For this review, take the finished solid that the model builds, in its own axes (mm). A direction names the side the tool comes from. Round coordinates to 2 decimals unless told otherwise and drop trailing zeros. Write each loop counter-clockwise with the first axis right and the second up, starting at its lowest first coordinate (ties: lowest second). Pieces come first, ordered by that corner, then holes. Notation, with made-up numbers: (-25, 50.5) -> (33, 50.5) arc R9 ccw to (33, 60.5) -> close; hole circle Ø5 at (12.5, 54.25). An arc over 180 degrees is marked (long way). Write each question's results on one line, items separated by ' | '. Start each with the question number.
Item 1: Tool access review of faces 5 (the cylindrical face through (0, -24, -36)), 6 (the flat face through (23, 0, -36)), 7 (the cylindrical face through (23.74, -18.524, -6.783)): name each direction out of +Z, -Z, +X, -X, +Y, -Y from which nothing blocks a thin tool from reaching the whole face with its end or side.
Item 2: Add section B-B (y = 10). State the section outline as (x, z) points.
Item 3: Clearance check with flat-ended pins moving along their axes: pin 1 (4 mm diameter, centred on x = 20, y = -19, fed in from -Z); pin 2 (23 mm diameter, centred on y = 6.5, z = -18.5, fed in from +X). State where each tip first meets the part, or that it passes through.
Item 4: Add section C-C (x = -22). State the section outline as (y, z) points.
Item 5: Add section A-A (z = -45). State the section outline as (x, y) points.
Item 6: Add section D-D (x = -3). State the section outline as (y, z) points.
Item 7: To check wall thickness, follow line 1 along Y through (x, z) = (24.8, -7); line 2 along Y through (x, z) = (24, -23); line 3 along Z through (x, y) = (23.7, -19.5). State the ranges of each line that lie inside material, in increasing order.
Item 8: The part is to be moulded in two halves that separate along X. For faces 1 (the flat face through (-2, -24, -60)), 2 (the flat face through (-25, 0, -30)), 3 (the flat face through (0, 23, -30)), 4 (the cylindrical face through (-7, -24, -31)), say which applies: +X half, -X half, draft (parallel to the pull), parting line (faces both ways), or undercut.
Autodesk Inventor part; units mm, degrees
ref_plane "YZ Plane" through (0, 0, 0) normal (1, 0, 0) x (0, 1, 0)
ref_plane "XZ Plane" through (0, 0, 0) normal (0, 1, 0) x (-1, 0, 0)
ref_plane "XY Plane" through (0, 0, 0) normal (0, 0, 1) x (1, 0, 0)
sketch "スケッチ1" plane through (0, 0, 0) normal (0, 0, 1) x (1, 0, 0)
  line L0 (-25, 25) -> (25, 25)
  line L1 (25, 25) -> (25, -25)
  line L2 (25, -25) -> (-25, -25)
  line L3 (-25, -25) -> (-25, 25)
  line L4 (-23, 23) -> (23, 23)
  line L5 (23, 23) -> (23, -23)
  line L6 (23, -23) -> (-23, -23)
  line L7 (-23, -23) -> (-23, 23)
  point P0 (0, 0)
  dimension "d0" = 23
  dimension "d1" = 25
  dimension "d2" = 50
  dimension "d3" = 46
  dimension "d4" = 46
  dimension "d5" = 50
  dimension "d6" = 23
  dimension "d7" = 25
extrude "押し出し1" add sketch "スケッチ1" against normal blind 60
sketch "スケッチ2" plane through (25, -25, 0) normal (1, 0, 0) x (0, 0, -1)
  line L0 (0, 50) -> (0, 0)
  line L1 (0, 0) -> (60, 0)
  circle A0 centre (15, 35) radius 2
  circle A1 centre (45, 29) radius 2
  point P0 (0, 25)
  dimension "d10" = 4
  dimension "d12" = 30
  dimension "d13" = 15
  dimension "d14" = 6
  dimension "d15" = 29
hole "穴1" at (25, 10, -15) at (25, 4, -45) direction (-1, 0, 0) diameter 4 end through all
sketch "スケッチ3" plane through (25, -25, 0) normal (1, 0, 0) x (0, 0, -1)
  circle A0 centre (15, 35) radius 2
  line L0 (0, 50) -> (60, 50)
  line L1 (8.5, 50) -> (21.5, 50)
  line L2 (21.5, 50) -> (21.5, 14.5)
  line L3 (8.5, 14.5) -> (8.5, 50)
  arc A1 (8.5, 14.5) -> (21.5, 14.5) centre (15, 14.5) ccw
  circle A2 centre (45, 29) radius 2
  point P0 (0, 25)
  dimension "d23" = 35.5
  dimension "d26" = 13
  dimension "d27" = 6.5
  dimension "d28" = 6.5
  dimension "d74" = 30
extrude "押し出し2" cut sketch "スケッチ3" against normal blind 2 contours L0 L2 A1 L3
sketch "スケッチ4" plane through (25, -25, 0) normal (1, 0, 0) x (0, 0, -1)
  line L0 (0, 50) -> (8.5, 50)
  line L1 (21.5, 50) -> (60, 50)
  circle A0 centre (7, 41.5) radius 1
  circle A1 centre (7, 5.5) radius 1
  circle A2 centre (23, 41.5) radius 1
  circle A3 centre (23, 5.5) radius 1
  arc A4 (8.5, 14.5) -> (21.5, 14.5) centre (15, 14.5) ccw
  point P0 (0, 25)
  dimension "d32" = 8.5
  dimension "d33" = 8.5
  dimension "d34" = 36
  dimension "d35" = 36
  dimension "d36" = 16
  dimension "d37" = 16
  dimension "d40" = 2
  dimension "d72" = 8
  dimension "d73" = 8
hole "穴2" at (25, 16.5, -7) at (25, 16.5, -23) at (25, -19.5, -7) at (25, -19.5, -23) direction (-1, 0, 0) diameter 2 depth 2 tip angle 118 counterbore diameter 4 counterbore depth 0.5
sketch "スケッチ5" plane through (-25, -25, 0) normal (0, -1, 0) x (1, 0, 0)
  line L0 (50, 0) -> (0, 0)
  line L1 (0, 0) -> (0, -60)
  circle A0 centre (25, -30) radius 5
  point P0 (25, 0)
  dimension "d48" = 25
  dimension "d49" = 30
  dimension "d50" = 10
hole "穴3" at (0, -25, -30) direction (0, 1, 0) diameter 10 depth 2 tip angle 118
sketch "スケッチ6" plane through (-25, -25, 0) normal (0, -1, 0) x (1, 0, 0)
  circle A0 centre (25, -30) radius 5
  line L0 (0, 0) -> (0, -60)
  circle A1 centre (25, -23) radius 1
  point P0 (25, 0)
  dimension "d58" = 2
  dimension "d60" = 7
  dimension "d61" = 25
hole "穴4" at (0, -25, -23) direction (0, 1, 0) diameter 2 depth 2 tip angle 118
pattern_circular "円形状パターン1" count 8 over 360 about axis through (0, -24, -30) along (0, -1, 0) of "穴4"
properties part number "Arm_Bracket_2"
Responses:
1) face 5: -Y | face 6: +Z, -Z | face 7: +X
2) outline: (-25, -60) -> (-23, -60) -> (-23, -17) -> (-25, -17) -> close; (-25, -13) -> (-23, -13) -> (-23, 0) -> (-25, 0) -> close; (23, -60) -> (25, -60) -> (25, -21.5) -> (23, -21.5) -> close; (23, -8.5) -> (25, -8.5) -> (25, 0) -> (23, 0) -> close
3) pin 1: passes through | pin 2: stops at x = 25
4) outline: (-25, -60) -> (-23, -60) -> (-23, 0) -> (-25, 0) -> close; (23, -60) -> (25, -60) -> (25, 0) -> (23, 0) -> close
5) outline: (-25, -25) -> (25, -25) -> (25, 2) -> (23, 2) -> (23, -23) -> (-23, -23) -> (-23, 2) -> (-25, 2) -> close; (-25, 6) -> (-23, 6) -> (-23, 23) -> (23, 23) -> (23, 6) -> (25, 6) -> (25, 25) -> (-25, 25) -> close
6) outline: (-25, -60) -> (-23, -60) -> (-23, -34) -> (-25, -34) -> close; (-25, -26) -> (-23, -26) -> (-23, 0) -> (-25, 0) -> close; (23, -60) -> (25, -60) -> (25, 0) -> (23, 0) -> close
7) line 1: y = -25 to -21.5, -17.5 to 14.5, 18.5 to 25 | line 2: y = -25 to -20.5, -18.5 to 15.5, 17.5 to 25 | line 3: z = -60 to -24, -22 to -8, -6 to 0
8) face 1: draft | face 2: -X half | face 3: undercut | face 4: undercut
